CAD build for the part. Positions are in the model's coordinates, mm. A direction names the side the tool comes from. Coordinates: 2 decimals unless noted, no trailing zeros. Order: outer loops, then holes, each group sorted by start corner. A loop starts at its lowest first (then second) coordinate and runs counter-clockwise, first axis right, second up. Notation, with made-up numbers: (-30, -9) - (-2, -9) arc R18 ccw to (-2, 26) - close; hole circle Ø7 at (-24.5, 29). An arc over 180 degrees is marked (long way). Use one line per item in the form item = value.
```python
from build123d import *

# Parameters (mm, degrees)
F1_DEPTH = 38
F2_R     = 5


with BuildPart() as f1:
    # F0 (on Top) → F1 (new body)
    with BuildSketch(Plane.XY):
        with BuildLine():
            Line((730.000074, 356.940193), (-639.999926, 356.940193))
            ThreePointArc((-639.999926, 356.940193), (-647.070994, 354.011261), (-649.999926, 346.940193))
            Line((-649.999926, 346.940193), (-649.999926, -259.059807))
            ThreePointArc((-649.999926, -259.059807), (-647.070994, -266.130875), (-639.999926, -269.059807))
            Line((-639.999926, -269.059807), (670.000074, -269.059807))
            Line((670.000074, -269.059807), (670.000074, 326.940193))
            Line((670.000074, 326.940193), (740.000074, 326.940193))
            Line((740.000074, 326.940193), (740.000074, 346.940193))
            ThreePointArc((740.000074, 346.940193), (737.071142, 354.011261), (730.000074, 356.940193))
        make_face()
    extrude(amount=F1_DEPTH)

    # F2
    f2_edges = [f1.edges().sort_by_distance(p)[0] for p in [
        (-649.999926, 43.940193, 38),
    ]]
    fillet(f2_edges, radius=F2_R)


solid = f1.part
```
Item 1: Drop a flat-ended pin along its axis: pin 1 (1 mm diameter, centred on y = 254.5, z = 10, fed in from +X). Give the stop position or say it passes through.
Derived:
pin_1 = 670
Item 2: Drill centre lines: line 1 (X direction, y = 56.5, z = 34); line 2 (X direction, y = 93, z = 32.5). Where is each one in solid material? Low to high. Write a range as [from, to].
Derived:
line_1 = [-649.9, 670]
line_2 = [-650, 670]
Item 3: Cut at B-B, the plane z = 11. Write the cut outline in (x, y).
Derived:
outline = (-650, -259.06) arc R10 ccw to (-640, -269.06) - (670, -269.06) - (670, 326.94) - (740, 326.94) - (740, 346.94) arc R10 ccw to (730, 356.94) - (-640, 356.94) arc R10 ccw to (-650, 346.94) - close
Item 4: Cut at A-A, the plane y = 61. Write the cut outline in (x, z), plus the area to 3 significant figures.
Derived:
outline = (-650, 0) - (670, 0) - (670, 38) - (-645, 38) arc R5 ccw to (-650, 33) - close
area = 50,200 mm²
Item 5: 3-axis set-ups, long thin cutter, end or side, ignore diameter. For faces 1 (the face through (55, 356.94, 16)), 2 (the face through (670, 25, 19)): which of +Z, -Z, +X, -X, +Y, -Y reach the whole face in a straight line?
Derived:
face_1 = +Z, -Z, +X, -X, +Y
face_2 = +Z, -Z, +X, -Y
